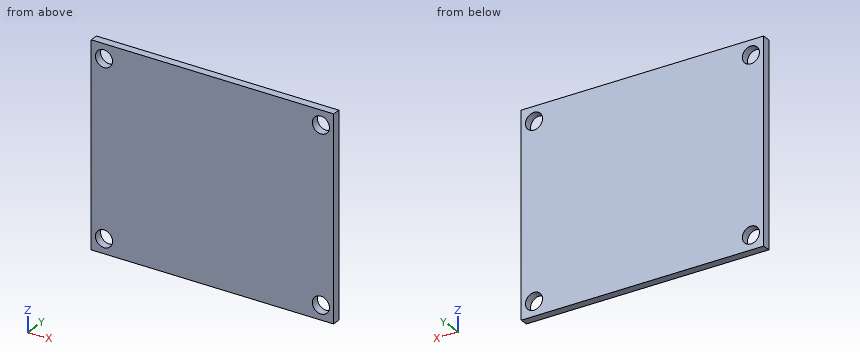
from build123d import *

# Parameters (mm, degrees)
SKETCH1_W            = 48.26
SKETCH1_H            = 40
BOSS_EXTRUDE1_DEPTH  = 1.5875
LPATTERN1_COUNT      = 2
LPATTERN1_PITCH      = 43.18
LPATTERN1_COUNT_DIR2 = 2
LPATTERN1_PITCH_DIR2 = 34.29


with BuildPart() as part:
    # Sketch1 → Boss-Extrude1 (new body)
    with BuildSketch(Plane(origin=(0, 0, 0), x_dir=(1, 0, 0), z_dir=(0, 1, 0))):
        with Locations((-18.638619051, 2.255163759)):
            Rectangle(SKETCH1_W, SKETCH1_H)
    extrude(amount=BOSS_EXTRUDE1_DEPTH)

    # Sketch9 → Clearance hole for 3MM screw (revolve, cut)
    with BuildSketch(Plane(origin=(-40.228619051, 1.5875, -19.400163759), x_dir=(0, 0, 1), z_dir=(1, 0, 0))):
        Polygon((0, 0), (0, 13.721463052), (1.7, 12.7), (1.7, 0), align=None)
    clearance_hole_for_3mm_screw = revolve(axis=Axis((-40.228619051, 7.9375, -19.400163759), (0, -1, 0)), mode=Mode.SUBTRACT)

    # LPattern1: Clearance hole for 3MM screw 2 × 2
    with Locations(*[(i * LPATTERN1_PITCH, 0, j * LPATTERN1_PITCH_DIR2) for i in range(LPATTERN1_COUNT) for j in range(LPATTERN1_COUNT_DIR2) if (i, j) != (0, 0)]):
        add(clearance_hole_for_3mm_screw, mode=Mode.SUBTRACT)


solid = part.part
Build history of the part. All positions in model axes, mm. Coordinates: 2 decimals unless noted, no trailing zeros. Order: outer loops, then holes, each group sorted by start corner. A loop starts at its lowest first (then second) coordinate and runs counter-clockwise, first axis right, second up. Notation, with made-up numbers: (-3.75, 3) - (41.25, 3) arc R14 cw to (41.25, 20) - close; hole circle Ø2 at (52, 55.25). An arc over 180 degrees is marked (long way). Write item = value, one per line. Start each with the question number.
1) Saw through at B-B on y = 0.95. Write the cut outline in (x, z), then the cut area to 3 significant figures.
2) Wall check: line 1 along X through (y, z) = (0.35, -19.5); line 2 along X through (y, z) = (1.5, 14); line 3 along Z through (x, y) = (-40, 1.05). Give the ranges that are in metal, low to high. Write a range as from..to.
3) Saw through at A-A on z = 15.5. Write the cut outline in (x, y), then the cut area to 3 significant figures.
From the geometry:
q1.outline = (-42.77, -22.26) - (5.49, -22.26) - (5.49, 17.74) - (-42.77, 17.74) - close; hole circle Ø3.4 at (-40.23, -19.4); hole circle Ø3.4 at (-40.23, 14.89); hole circle Ø3.4 at (2.95, -19.4); hole circle Ø3.4 at (2.95, 14.89)
q1.area = 1,890 mm^2
q2.line_1 = -42.77..-41.93, -38.53..1.25, 4.65..5.49
q2.line_2 = -42.77..-41.68, -38.78..1.5, 4.4..5.49
q2.line_3 = -22.26..-21.08, -17.72..13.21, 16.57..17.74
q3.outline = (-42.77, 0) - (-41.82, 0) - (-41.82, 1.59) - (-42.77, 1.59) - close; (-38.64, 0) - (1.36, 0) - (1.36, 1.59) - (-38.64, 1.59) - close; (4.54, 0) - (5.49, 0) - (5.49, 1.59) - (4.54, 1.59) - close
q3.area = 66.5 mm^2
